Source: CAD feature listing. Evaluate the final solid. Frame: model axes, mm. Face numbers are marked on the shaded views. A direction names the side the tool comes from. Coordinates: 2 decimals unless noted, no trailing zeros. Order: outer loops, then holes, each group sorted by start corner. A loop starts at its lowest first (then second) coordinate and runs counter-clockwise, first axis right, second up.
Item 1: Contact query for flat-ended pins moving along their axis: P1, Ø1.5, axis at y = -11.5, z = -1, coming from the -X side; P2, Ø2.5, axis at y = 1.5, z = 1.5, coming from the +X side; P3, Ø3, axis at y = 19, z = -1, coming from the +X side. Output: stop coordinate, or through.
Item 2: Section D-D on y = -22. Return the cut outline in (x, z).
Item 3: Section A-A on z = 1. Return the cut outline in (x, y).
Item 4: Section C-C on x = 10. Return the cut outline in (y, z).
Item 5: Reachability of the marked faces 1, 2 and 3 from +Z, -Z, +X, -X, +Y, -Y: full face, straight path, thin tool, end or side. Return the list, or none.
Item 6: Section B-B on y = 4. Return the cut outline in (x, z).
Item 7: Mould query, pull axis Y, two halves, no side actions, for the marked faces 4, 5, 6 and 7. Classes: released by +Y, released by -Y, zero draft, split by the parting line, or undercut.
Item 8: Ray query, line 1 (Y direction, x = -10, z = 2.75); line 2 (Y direction, x = -10, z = -0.75); line 3 (X direction, y = -12, z = 1). Return the intervals inside material, ascending.
from build123d import *

# Parameters (mm, degrees)
F0_W          = 52
F0_H          = 31
F1_DEPTH      = 3
F2_W          = 10
F2_H          = 31
F3_DEPTH      = 5
F4_SIZE       = 3
F5_R          = 2.9
F6_DEPTH      = 4
F7_W          = 90
F7_H          = 52
F8_DEPTH      = 2
F8_DEPTH_BACK = 1
F9_DEPTH      = 1
F10_DEPTH     = 2
F11_R         = 20
F12_R         = 1.5
F13_DEPTH     = 25
F14_R         = 1.5
F15_DEPTH     = 25
F17_DEPTH     = 25
F18_W         = 10
F18_H         = 31
F19_DEPTH     = 25
F20_W         = 10
F20_H         = 20
F21_DEPTH     = 25
F22_W         = 10
F22_H         = 20
F23_DEPTH     = 25
F24_R         = 2


with BuildPart() as f1:
    # F0 (on Top) → F1 (new body)
    with BuildSketch(Plane.XY):
        Rectangle(F0_W, F0_H)
    extrude(amount=-F1_DEPTH)

    # F2 (on face) → F3 (join)
    with BuildSketch(Plane.XY):
        with Locations((21, 0)):
            Rectangle(F2_W, F2_H)
        with Locations((-21, 0)):
            Rectangle(F2_W, F2_H)
    extrude(amount=F3_DEPTH)

    # F4
    f4_edges = [f1.edges().sort_by_distance(p)[0] for p in [
        (-16, 0, 5),
        (16, 0, 5),
    ]]
    chamfer(f4_edges, length=F4_SIZE)

    # F5 (on face) → F6 (join)
    with BuildSketch(Plane.XY):
        with Locations((-10, 0)):
            Circle(F5_R)
        with Locations((10, 0)):
            Circle(F5_R)
    extrude(amount=F6_DEPTH)

    # F7 (on face) → F8 (join, two sides)
    with BuildSketch(Plane(origin=(0, 0, -3), x_dir=(1, 0, 0), z_dir=(0, 0, -1))) as f8_sk:
        Rectangle(F7_W, F7_H)
    extrude(amount=F8_DEPTH)
    extrude(f8_sk.sketch, amount=-F8_DEPTH_BACK)

    # F9 (add): a face of the model
    f9_faces = [f1.faces().sort_by_distance(p)[0] for p in [
        (43.9605770832, 0, -2),
    ]]
    extrude(f9_faces, amount=F9_DEPTH)

    # F10 (cut): a face of the model
    f10_faces = [f1.faces().sort_by_distance(p)[0] for p in [
        (0, 0, -5),
    ]]
    extrude(f10_faces, amount=-F10_DEPTH, mode=Mode.SUBTRACT)

    # F11
    f11_edges = [f1.edges().sort_by_distance(p)[0] for p in [
        (45, 26, -2),
        (-45, 26, -2),
        (-45, -26, -2),
        (45, -26, -2),
    ]]
    fillet(f11_edges, radius=F11_R)

    # F12 (on face) → F13 (cut)
    with BuildSketch(Plane.XY.offset(4)):
        with Locations((-10, 0)):
            Circle(F12_R)
    extrude(amount=-F13_DEPTH, mode=Mode.SUBTRACT)

    # F14 (on face) → F15 (cut)
    with BuildSketch(Plane.XY.offset(4)):
        with Locations((10, 0)):
            Circle(F14_R)
    extrude(amount=-F15_DEPTH, mode=Mode.SUBTRACT)

    # F16 (on face) → F17 (cut)
    with BuildSketch(Plane.XY.offset(-1)):
        with BuildLine():
            Line((26, 15.3868599666), (26, -15.3868599666))
            ThreePointArc((26, -15.3868599666), (32.0828754441, -12.0192024052), (34.5, -5.5))
            Line((34.5, -5.5), (34.5, 5.5))
            ThreePointArc((34.5, 5.5), (32.0828754441, 12.0192024052), (26, 15.3868599666))
        make_face()
        with BuildLine():
            ThreePointArc((-34.5, -5.5), (-32.0828754441, -12.0192024052), (-26, -15.3868599666))
            Line((-26, -15.3868599666), (-26, 15.3868599666))
            ThreePointArc((-26, 15.3868599666), (-32.0828754441, 12.0192024052), (-34.5, 5.5))
            Line((-34.5, 5.5), (-34.5, -5.5))
        make_face()
    extrude(amount=-F17_DEPTH, mode=Mode.SUBTRACT)

    # F18 (on face) → F19 (cut)
    with BuildSketch(Plane.XY):
        Rectangle(F18_W, F18_H)
    extrude(amount=-F19_DEPTH, mode=Mode.SUBTRACT)

    # F20 (on face) → F21 (cut)
    with BuildSketch(Plane.XY.offset(5)):
        with Locations((26, 0)):
            Rectangle(F20_W, F20_H)
    extrude(amount=-F21_DEPTH, mode=Mode.SUBTRACT)

    # F22 (on face) → F23 (cut)
    with BuildSketch(Plane.XY.offset(5)):
        with Locations((-26, 0)):
            Rectangle(F22_W, F22_H)
    extrude(amount=-F23_DEPTH, mode=Mode.SUBTRACT)

    # F24
    f24_edges = [f1.edges().sort_by_distance(p)[0] for p in [
        (21, 10, 1),
        (21, -10, 1),
        (-21, 10, 1),
        (-21, -10, 1),
        (-26, -10, 1),
        (-26, 10, 1),
        (26, 10, 1),
        (26, -10, 1),
    ]]
    fillet(f24_edges, radius=F24_R)


solid = f1.part
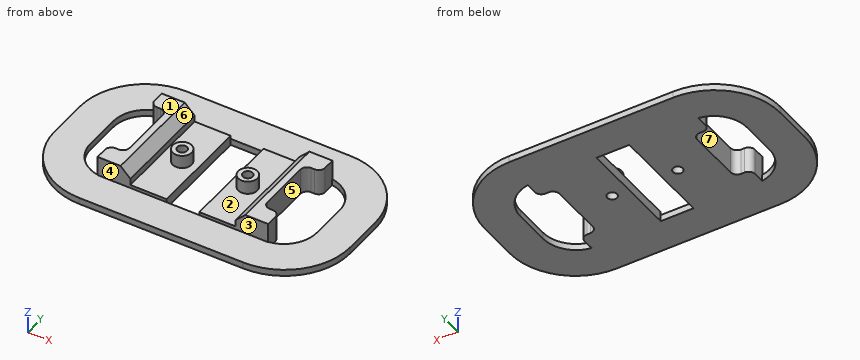
Answer list:
1. P1: stops at x = -44.43
1. P2: stops at x = 21
1. P3: stops at x = 41.36
2. outline: (-37, -3) - (37, -3) - (37, -1) - (-37, -1) - close
3. outline: (-26, -15.5) - (-16, -15.5) - (-16, 15.5) - (-26, 15.5) - (-26, 12) arc R2 ccw to (-24, 10) - (-23, 10) arc R2 cw to (-21, 8) - (-21, -8) arc R2 cw to (-23, -10) - (-24, -10) arc R2 ccw to (-26, -12) - close; circle Ø5.8 at (-10, 0); circle Ø5.8 at (10, 0); (16, -15.5) - (26, -15.5) - (26, -12) arc R2 ccw to (24, -10) - (23, -10) arc R2 cw to (21, -8) - (21, 8) arc R2 cw to (23, 10) - (24, 10) arc R2 ccw to (26, 12) - (26, 15.5) - (16, 15.5) - close; hole circle Ø3 at (-10, 0); hole circle Ø3 at (10, 0)
4. outline: (-26, -3) - (-1.5, -3) - (-1.5, 4) - (-2.9, 4) - (-2.9, 0) - (-15.5, 0) - (-15.5, -1) - (-26, -1) - close; (1.5, -3) - (26, -3) - (26, -1) - (15.5, -1) - (15.5, 0) - (2.9, 0) - (2.9, 4) - (1.5, 4) - close
5. face 1: +Z, +X, -X, +Y, -Y
5. face 2: +Z
5. face 3: +Z, +X, -X, -Y
6. outline: (-45, -3) - (-34.5, -3) - (-34.5, -1) - (-45, -1) - close; (-21, -3) - (-5, -3) - (-5, 0) - (-16, 0) - (-16, 2) - (-19, 5) - (-21, 5) - close; (5, -3) - (21, -3) - (21, 5) - (19, 5) - (16, 2) - (16, 0) - (5, 0) - close; (34.5, -3) - (45, -3) - (45, -1) - (34.5, -1) - close
7. face 4: released by -Y
7. face 5: undercut
7. face 6: zero draft
7. face 7: undercut
8. line 1: y = -2.9 to -1.5, 1.5 to 2.9
8. line 2: y = -15.5 to -1.5, 1.5 to 15.5
8. line 3: x = -26 to -16, 16 to 26
